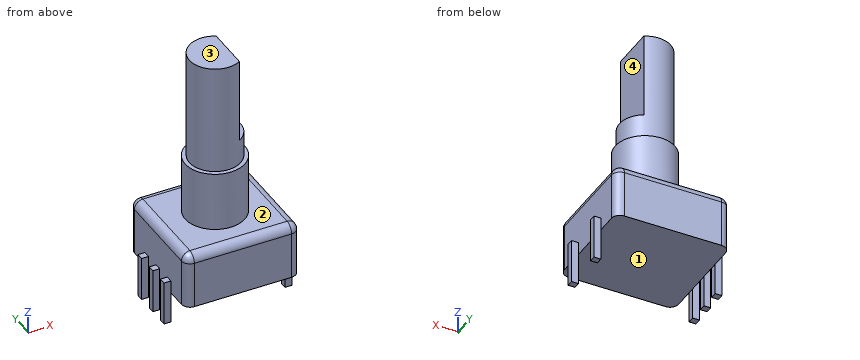
```python
from build123d import *

# Parameters (mm, degrees)
SKETCH_W      = 13.4
SKETCH_H      = 12.5
PAD_DEPTH     = 6.5
SKETCH001_W   = 0.8
SKETCH001_H   = 0.8
SKETCH001_H_2 = 0.76989
PAD001_DEPTH  = 5.2
SKETCH002_R   = 3.5
PAD002_DEPTH  = 7
SKETCH003_R   = 3
PAD003_DEPTH  = 13
POCKET_DEPTH  = 10
FILLET_R      = 1


with BuildPart() as part:
    # Sketch → Pad (new body)
    with BuildSketch(Plane.XY):
        with Locations((7.5, -2.5)):
            Rectangle(SKETCH_W, SKETCH_H)
    extrude(amount=PAD_DEPTH)

    # Sketch001 (on DatumPlane) → Pad001 (join)
    with BuildSketch(Plane(origin=(0, 0, 1.5), x_dir=(1, 0, 0), z_dir=(0, 0, -1))):
        with Locations((0.4, 5)):
            Rectangle(SKETCH001_W, SKETCH001_H)
        with Locations((0.4, 2.5)):
            Rectangle(SKETCH001_W, SKETCH001_H)
        with Locations((0.4, 0)):
            Rectangle(SKETCH001_W, SKETCH001_H)
        with Locations((14.6, 5)):
            Rectangle(SKETCH001_W, SKETCH001_H_2)
        with Locations((14.6, 0)):
            Rectangle(SKETCH001_W, SKETCH001_H_2)
    extrude(amount=PAD001_DEPTH)

    # Sketch002 (on Face5 of Pad001) → Pad002 (join)
    with BuildSketch(Plane.XY.offset(6.5)):
        with Locations((7.5, -2.5)):
            Circle(SKETCH002_R)
    extrude(amount=PAD002_DEPTH)

    # Sketch003 (on Face38 of Pad002) → Pad003 (join)
    with BuildSketch(Plane.XY.offset(13.5)):
        with Locations((7.5, -2.5)):
            Circle(SKETCH003_R)
    extrude(amount=PAD003_DEPTH)

    # Sketch004 (on Face40 of Pad003) → Pocket (cut)
    with BuildSketch(Plane.XY.offset(26.5)):
        with BuildLine():
            Line((9, 0.098076), (9, -5.098076))
            ThreePointArc((9, -5.098076), (10.5, -2.5), (9, 0.098076))
        make_face()
    extrude(amount=-POCKET_DEPTH, mode=Mode.SUBTRACT)

    # Fillet
    fillet_edges = [part.edges().sort_by_distance(p)[0] for p in [
        (0.8, 3.75, 3.25),
        (7.5, 3.75, 6.5),
        (0.8, -2.5, 6.5),
        (14.2, -2.5, 6.5),
        (14.2, 3.75, 3.25),
        (0.8, -8.75, 3.25),
        (7.5, -8.75, 6.5),
        (14.2, -8.75, 3.25),
    ]]
    fillet(fillet_edges, radius=FILLET_R)


solid = part.part
```
Work out the finished part from the listing and answer in its coordinate system (mm). Face numbers are marked on the shaded views. A direction names the side the tool comes from. Round coordinates to 2 decimals unless told otherwise and drop trailing zeros. Loops run counter-clockwise (first coordinate to the right, second up) from the corner with the lowest first, then second, coordinate; pieces in that order, holes last. Notation, with made-up numbers: M -12.5,-15 L 33.5,-15 A23 ccw 33.5,0 Z; hole C 20,37 d11. An arc over 180 degrees is marked long. Use CSV: the item, a comma, the result in double quotes.
Q1. A tool of negligible diameter and unlimited length cuts with its end or side. For the marked faces 1, 2, 3 and 4, from which of +Z, -Z, +X, -X, +Y, -Y can it reach the whole face along a straight path? Write none if from no direction.
Determined:
face 1,"-Z, +Y, -Y"
face 2,"+Z"
face 3,"+Z, +X, -X, +Y, -Y"
face 4,"+Z, +X, +Y, -Y"
Q2. Consider L1, parallel to Z at x = 4, y = 1; L2, parallel to X at y = -1.25, z = 1.5; L3, parallel to Z at x = 7.5, y = -3.5. Determine where each line is inside the solid, lowest interval first.
Determined:
L1,"0 to 6.5"
L2,"0.8 to 14.2"
L3,"0 to 26.5"
Q3. Section C-C, the plane x = 7.5 is taken. Determine the outline of the cut face in (y, z), then the cut area to 3 significant figures.
Determined:
outline,"M -8.75,0 L 3.75,0 L 3.75,5.5 A1 ccw 2.75,6.5 L 1,6.5 L 1,13.5 L 0.5,13.5 L 0.5,26.5 L -5.5,26.5 L -5.5,13.5 L -6,13.5 L -6,6.5 L -7.75,6.5 A1 ccw -8.75,5.5 Z"
area,"208 mm2"
Q4. Section B-B, the plane y = -2.5 is taken. Determine the outline of the cut face in (x, z), then the cut area to 3 significant figures.
Determined:
outline,"M 0,-3.7 L 0.8,-3.7 L 0.8,0 L 14.2,0 L 14.2,5.5 A1 ccw 13.2,6.5 L 11,6.5 L 11,13.5 L 10.5,13.5 L 10.5,16.5 L 9,16.5 L 9,26.5 L 4.5,26.5 L 4.5,13.5 L 4,13.5 L 4,6.5 L 1.8,6.5 A1 ccw 0.8,5.5 L 0.8,1.5 L 0,1.5 Z"
area,"203 mm2"
Q5. Section A-A, the plane z = -0.5 is taken. Determine the outline of the cut face in (x, y).
Determined:
outline,"M 0,-5.4 L 0.8,-5.4 L 0.8,-4.6 L 0,-4.6 Z; M 0,-2.9 L 0.8,-2.9 L 0.8,-2.1 L 0,-2.1 Z; M 0,-0.4 L 0.8,-0.4 L 0.8,0.4 L 0,0.4 Z; M 14.2,-5.38 L 15,-5.38 L 15,-4.62 L 14.2,-4.62 Z; M 14.2,-0.38 L 15,-0.38 L 15,0.38 L 14.2,0.38 Z"
Q6. Section D-D, the plane z = 13 is taken. Determine the outline of the cut face in (x, y).
Determined:
outline,"C 7.5,-2.5 d7"
Q7. Each of these flat-tipped pins is pushed along its axis until it touches: pin 1 (2.5 mm diameter, centred on y = -1.5, z = 24, fed in from +X); pin 2 (1.5 mm diameter, centred on y = -7, z = 6.5, fed in from -X); pin 3 (1.6 mm diameter, centred on x = 10, y = -3, fed in from +Z). Where does it stop, or does it pass through?
Determined:
pin 1,"x = 9"
pin 2,"x = 0.83"
pin 3,"z = 16.5"
